Part model, mm, in its own coordinate system. A direction names the side the tool comes from. Round coordinates to 2 decimals unless told otherwise and drop trailing zeros. Order: outer loops, then holes, each group sorted by start corner. A loop starts at its lowest first (then second) coordinate and runs counter-clockwise, first axis right, second up. Notation, with made-up numbers: (67, -4) - (84, -4) arc R19 cw to (84, 14) - close; hole circle Ø1 at (-16.75, -33.5). An arc over 180 degrees is marked (long way). Return JSON: item names as keys, results as strings. Group by question number.
Item 1: Saw through at A-A on z = 5.5. List the corners of the cut face in (x, y) (1 decimal).
Item 2: Saw through at C-C on x = 3. List the corners of the cut face in (y, z), and give its area (3 significant figures).
Item 3: Probe probe 1 along Z at (x, y) = (-9.5, -5); probe 2 along X at (y, z) = (-7, 2) (3 decimals); probe 3 along X at (y, z) = (-5.75, 2.5) (3 decimals). List the from-to ranges inside material, lowest first.
Item 4: Two-plate mould, pull along X, no slides. Class faces 4 (the face through (-1.38, -6.2, 37.92)), 5 (the face through (0, 0, 8)), 6 (the face through (0, 0, 50.8)): released by +X, released by -X, zero draft, split by the parting line, or undercut.
Item 5: Saw through at D-D on z = 22.5. List the corners of the cut face in (x, y) (1 decimal), and give its area (3 significant figures).
Item 6: Drop flat-ended pins along their axis: pin 1 (9.5 mm diameter, centred on y = 5, z = 10, fed in from +X); pin 2 (1 mm diameter, centred on y = -2, z = 8, fed in from +X); pin 3 (6 mm diameter, centred on y = 8.5, z = 40, fed in from +X); pin 4 (10 mm diameter, centred on x = 1.5, y = 8, fed in from +Z). Give the stop position or say it passes through.
Item 7: Tool access for faces 1 (the face through (-6, 0, 0)), 2 (the face through (4.696, 0.2, 15.567)), 3 (the face through (6, -3, 25.4)): list every direction of +Z, -Z, +X, -X, +Y, -Y with a clear straight run to the whole face (end or side of a thin tool).
```python
from build123d import *

# Parameters (mm, degrees)
F0_R     = 14.2875
F1_DEPTH = 25.4
F2_R     = 6.35
F3_DEPTH = 25.4
F7_DEPTH = 9.525


with BuildPart() as f1:
    # F0 (on Top) → F1 (new body)
    with BuildSketch(Plane.XY):
        Circle(F0_R)
    extrude(amount=F1_DEPTH)

    # F2 (on face) → F3 (join)
    with BuildSketch(Plane.XY.offset(25.4)):
        Circle(F2_R)
    extrude(amount=F3_DEPTH)

    # F6 (on Right) → F7 (cut)
    with BuildSketch(Plane.YZ):
        Polygon((-14.2875, 0), (-11.1125, 0), (11.103606, 0), (14.2875, 0), (14.2875, 11.79217), (-14.2875, 19.448818), align=None)
    extrude(amount=F7_DEPTH, mode=Mode.SUBTRACT)


solid = f1.part
```
Filled in:
{
 "1": {"outline": "(0, -14.3) - (0, 14.3) arc R14.3 ccw to start; (9.5, -10.6) arc R14.3 ccw to (9.5, 10.6) - close"},
 "2": {"outline": "(-13.97, 19.36) - (13.97, 11.88) - (13.97, 25.4) - (5.6, 25.4) - (5.6, 50.8) - (-5.6, 50.8) - (-5.6, 25.4) - (-13.97, 25.4) - close", "area": "558 mm^2"},
 "3": {"probe 1": "z = 0 to 25.4", "probe 2": "x = -12.455 to 0, 9.525 to 12.455", "probe 3": "x = -13.079 to 0, 9.525 to 13.079"},
 "4": {"face 4": "split by the parting line", "face 5": "undercut", "face 6": "zero draft"},
 "5": {"outline": "circle Ø28.6 at (0, 0)", "area": "641 mm^2"},
 "6": {"pin 1": "stops at x = 14.29", "pin 2": "stops at x = 14.21", "pin 3": "stops at x = 3.17", "pin 4": "stops at z = 50.8"},
 "7": {"face 1": "-Z, +X, -X, +Y, -Y", "face 2": "-Z, -Y", "face 3": "+Z"}
}
